Geometry check sheet. Reference: the model listing, model coordinates, mm. Face numbers are marked on the shaded views. A direction names the side the tool comes from. Round coordinates to 2 decimals unless told otherwise and drop trailing zeros. Order: outer loops, then holes, each group sorted by start corner. A loop starts at its lowest first (then second) coordinate and runs counter-clockwise, first axis right, second up.
(1) Sectioned sample at C-C (y = -0.25). Record the boundary of the cut face in (x, z), plus the area to 3 significant figures.
(2) Go/stop test with a flat-tipped pin: pin 1 (6 mm diameter, centred on x = 6.5, z = -0.5, fed in from -Y). Record where the tip stops, or that it passes through.
(3) Sectioned sample at D-D (x = 6.5). Record the boundary of the cut face in (y, z).
(4) Sectioned sample at B-B (x = 10.25). Record the boundary of the cut face in (y, z), plus the area to 3 significant figures.
(5) Release check for a two-part mould opening along Z. For the marked faces 3, 4, 5 and 6 record: +Z half, -Z half, draft (parallel to the pull), parting line (faces both ways), or undercut.
(6) Set-up check for the marked faces 1 and 2: record each of +Z, -Z, +X, -X, +Y, -Y from which the full face is reachable in a straight line by a thin tool's end or side.
(7) Sectioned sample at A-A (y = -8.6). Record the boundary of the cut face in (x, z), plus the area to 3 significant figures.
(8) Material ranges on line 1 along Z through (x, y) = (2.25, -2.5); line 2 along Y through (x, z) = (9, 0); line 3 along Y through (x, z) = (6.5, 4.2), recorded low to high.
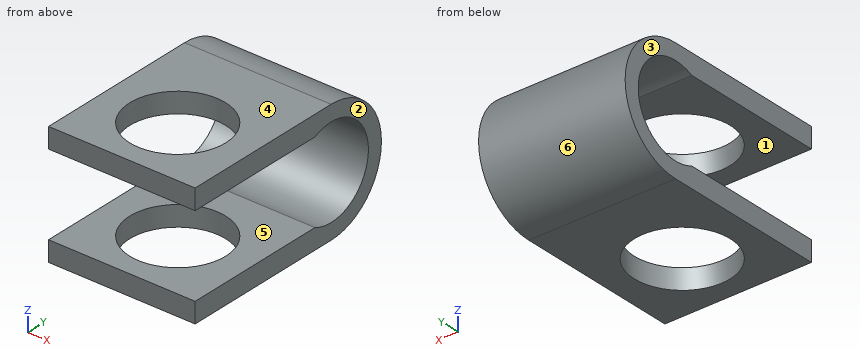
from build123d import *

# Parameters (mm, degrees)
BOSS_EXTRUDE1_DEPTH = 13
SKETCH2_R           = 4.25
CUT_EXTRUDE1_DEPTH  = 23.33383084


with BuildPart() as part:
    # Sketch1 → Boss-Extrude1 (new body)
    with BuildSketch(Plane(origin=(0, 0, 0), x_dir=(0, 0, -1), z_dir=(1, 0, 0))):
        with BuildLine():
            Line((5.4, 0), (5.4, -14.6))
            Line((5.4, -14.6), (3.6, -14.6))
            Line((3.6, -14.6), (3.6, -1.743559577))
            ThreePointArc((3.6, -1.743559577), (0, 4), (-3.6, -1.743559577))
            Line((-3.6, -1.743559577), (-3.6, -14.6))
            Line((-3.6, -14.6), (-5.4, -14.6))
            Line((-5.4, -14.6), (-5.4, 0))
            ThreePointArc((-5.4, 0), (0, 5.4), (5.4, 0))
        make_face()
    extrude(amount=BOSS_EXTRUDE1_DEPTH)

    # Sketch2 → Cut-Extrude1 (cut, through all)
    with BuildSketch(Plane.XY.offset(5.4)):
        with Locations((6.5, -8.6)):
            Circle(SKETCH2_R)
    extrude(amount=-CUT_EXTRUDE1_DEPTH, mode=Mode.SUBTRACT)


solid = part.part
Answer below:
1. outline: (0, -5.4) - (13, -5.4) - (13, -3.99) - (0, -3.99) - close; (0, 3.99) - (13, 3.99) - (13, 5.4) - (0, 5.4) - close
1. area: 36.6 mm2
2. pin 1: stops at y = 1.94
3. outline: (-14.6, -5.4) - (-12.85, -5.4) - (-12.85, -3.6) - (-14.6, -3.6) - close; (-14.6, 3.6) - (-12.85, 3.6) - (-12.85, 5.4) - (-14.6, 5.4) - close; (-4.35, -5.4) - (0, -5.4) arc R5.4 ccw to (0, 5.4) - (-4.35, 5.4) - (-4.35, 3.6) - (-1.74, 3.6) arc R4 cw (long way) to (-1.74, -3.6) - (-4.35, -3.6) - close
4. outline: (-14.6, -5.4) - (-10.6, -5.4) - (-10.6, -3.6) - (-14.6, -3.6) - close; (-14.6, 3.6) - (-10.6, 3.6) - (-10.6, 5.4) - (-14.6, 5.4) - close; (-6.6, -5.4) - (0, -5.4) arc R5.4 ccw to (0, 5.4) - (-6.6, 5.4) - (-6.6, 3.6) - (-1.74, 3.6) arc R4 cw (long way) to (-1.74, -3.6) - (-6.6, -3.6) - close
4. area: 57.9 mm2
5. face 3: draft
5. face 4: +Z half
5. face 5: undercut
5. face 6: parting line
6. face 1: +X, -X, -Y
6. face 2: +Z, -Z, +X, +Y, -Y
7. outline: (0, -5.4) - (2.25, -5.4) - (2.25, -3.6) - (0, -3.6) - close; (0, 3.6) - (2.25, 3.6) - (2.25, 5.4) - (0, 5.4) - close; (10.75, -5.4) - (13, -5.4) - (13, -3.6) - (10.75, -3.6) - close; (10.75, 3.6) - (13, 3.6) - (13, 5.4) - (10.75, 5.4) - close
7. area: 16.2 mm2
8. line 1: z = -5.4 to -3.6, 3.6 to 5.4
8. line 2: y = 4 to 5.4
8. line 3: y = -14.6 to -12.85, -4.35 to 3.39
